Model file for the job. Use its own axes, mm. A direction names the side the tool comes from. Round coordinates to 2 decimals unless told otherwise and drop trailing zeros. Loops run counter-clockwise (first coordinate to the right, second up) from the corner with the lowest first, then second, coordinate; pieces in that order, holes last. Notation, with made-up numbers: M -12,29 L -2,29 A22 cw -2,62 Z; hole C 14,72 d6. An arc over 180 degrees is marked long. Use a Markdown table: item, result. Add a question column.
Q1. Probe line 1 (X direction, y = 22.5, z = -2); line 2 (Y direction, x = -21, z = 6.5); line 3 (Z direction, x = 8.5, y = 35). List the from-to ranges inside material, lowest first. Write a range as from..to.
Q2. Mould opens along X. For faces 1 (the face through (-21, 20, 5)), 2 (the face through (20, 40, 5)), 3 (the face through (-43.872, 10.14, 9.614)) say: +X half, -X half, draft (parallel to the pull), parting line (faces both ways), or undercut.
Q3. Cut at A-A (y = 53.5). Give the cut face in (x, z).
Q4. Cut at D-D (y = 37). Give the cut face in (x, z).
Q5. Cut at B-B (x = 37.5). Give the cut face in (y, z), plus the area to 3 significant figures.
Q6. Cut at C-C (z = -18). Give the cut face in (x, y), plus the area to 3 significant figures.
Q7. Pin check, flat tips, straight feed: pin 1 (1 mm diameter, centred on x = -36, y = 13.5, fed in from +Z) (3 decimals); pin 2 (8 mm diameter, centred on y = 29.5, z = -2, fed in from -X); pin 3 (25 mm diameter, centred on x = -6, z = 12, fed in from +Y). Stop position of each tip, or through.
Q8. Tool access for faces 4 (the face through (40, 55, -10)), 5 (the face through (60, 30, 0)), 6 (the face through (-21, 40, -20)): list every direction of +Z, -Z, +X, -X, +Y, -Y with a clear straight run to the whole face (end or side of a thin tool).
from build123d import *

# Parameters (mm, degrees)
SKETCH1_W           = 120
SKETCH1_H           = 60
BOSS_EXTRUDE1_DEPTH = 20
SKETCH2_W           = 120
SKETCH2_H           = 10
BOSS_EXTRUDE2_DEPTH = 40
CHAMFER1_SIZE       = 20
FILLET1_R           = 25
SKETCH4_W           = 40
SKETCH4_H           = 50
BOSS_EXTRUDE5_DEPTH = 40
SKETCH5_W           = 40
SKETCH5_H           = 30
CUT_EXTRUDE1_DEPTH  = 10
SKETCH6_R           = 10
CUT_EXTRUDE2_DEPTH  = 79.102496759


with BuildPart() as part:
    # Sketch1 → Boss-Extrude1 (new body)
    with BuildSketch(Plane(origin=(0, 0, 0), x_dir=(1, 0, 0), z_dir=(0, 1, 0))):
        Rectangle(SKETCH1_W, SKETCH1_H)
    extrude(amount=BOSS_EXTRUDE1_DEPTH)

    # Sketch2 → Boss-Extrude2 (add)
    with BuildSketch(Plane(origin=(0, 20, 0), x_dir=(1, 0, 0), z_dir=(0, 1, 0))):
        with Locations((0, 25)):
            Rectangle(SKETCH2_W, SKETCH2_H)
    extrude(amount=BOSS_EXTRUDE2_DEPTH)

    # Chamfer1
    chamfer1_edges = [part.edges().sort_by_distance(p)[0] for p in [
        (-60, 60, -25),
    ]]
    chamfer(chamfer1_edges, length=CHAMFER1_SIZE)

    # Fillet1
    fillet1_edges = [part.edges().sort_by_distance(p)[0] for p in [
        (-60, 10, 30),
    ]]
    fillet(fillet1_edges, radius=FILLET1_R)

    # Sketch4 → Boss-Extrude5 (add)
    with BuildSketch(Plane(origin=(0, 20, 0), x_dir=(1, 0, 0), z_dir=(0, 1, 0))):
        with Locations((40, -5)):
            Rectangle(SKETCH4_W, SKETCH4_H)
    extrude(amount=BOSS_EXTRUDE5_DEPTH)

    # Sketch5 → Cut-Extrude1 (cut)
    with BuildSketch(Plane(origin=(0, 60, 0), x_dir=(1, 0, 0), z_dir=(0, 1, 0))):
        with Locations((40, -5)):
            Rectangle(SKETCH5_W, SKETCH5_H)
    extrude(amount=-CUT_EXTRUDE1_DEPTH, mode=Mode.SUBTRACT)

    # Sketch6 → Cut-Extrude2 (cut, through all)
    with BuildSketch(Plane(origin=(0, 20, 0), x_dir=(1, 0, 0), z_dir=(0, 1, 0))):
        with Locations(Location((-35, -5, 0), (0, 0, 270))):
            Circle(SKETCH6_R)
    extrude(amount=-CUT_EXTRUDE2_DEPTH, mode=Mode.SUBTRACT)


solid = part.part
Checked values:
| question | item | result |
|---|---|---|
| 1 | line 1 | x = 20..60 |
| 1 | line 2 | y = 0..20 |
| 1 | line 3 | z = -30..-20 |
| 2 | face 1 | draft |
| 2 | face 2 | -X half |
| 2 | face 3 | undercut |
| 3 | outline | M -46.5,-30 L 60,-30 L 60,-10 L 20,-10 L 20,-20 L -46.5,-20 Z; M 20,20 L 60,20 L 60,30 L 20,30 Z |
| 4 | outline | M -60,-30 L 60,-30 L 60,30 L 20,30 L 20,-20 L -60,-20 Z |
| 5 | outline | M 0,-30 L 60,-30 L 60,-10 L 50,-10 L 50,20 L 60,20 L 60,30 L 0,30 Z |
| 5 | area | 3,300 mm^2 |
| 6 | outline | M -60,0 L 60,0 L 60,60 L 20,60 L 20,20 L -60,20 Z |
| 6 | area | 4,000 mm^2 |
| 7 | pin 1 | stops at z = 29.995 |
| 7 | pin 2 | stops at x = 20 |
| 7 | pin 3 | stops at y = 20 |
| 8 | face 4 | +X, -X, +Y |
| 8 | face 5 | +Z, -Z, +X, +Y, -Y |
| 8 | face 6 | +Z, -X, +Y |
